Can you work these out from the model? Positions are in its coordinate system, mm. A direction names the side the tool comes from. Give positions to 0.01 mm unless a question says otherwise; leave off trailing zeros. Loops run counter-clockwise (first coordinate to the right, second up) from the corner with the lowest first, then second, coordinate; pieces in that order, holes last. Notation, with made-up numbers: M 5.5,7.5 L 11.5,7.5 A25 cw 11.5,44.5 Z; hole C 50,-31.75 d6. An arc over 180 degrees is marked long. Answer as a JSON object with one key per item and string values.
```python
from build123d import *

# Parameters (mm, degrees)
SKETCH1_W           = 154
SKETCH1_H           = 51
SKETCH1_R           = 1.7
BOSS_EXTRUDE1_DEPTH = 4
SKETCH2_W           = 127
SKETCH2_H           = 28
BOSS_EXTRUDE2_DEPTH = 10


with BuildPart() as part:
    # Sketch1 → Boss-Extrude1 (new body)
    with BuildSketch(Plane(origin=(0, 0, 0), x_dir=(1, 0, 0), z_dir=(0, 1, 0))):
        with Locations((77, 25.5)):
            Rectangle(SKETCH1_W, SKETCH1_H)
        with Locations(Location((77, 25.5, 0), (0, 0, 270))):
            Circle(SKETCH1_R, mode=Mode.SUBTRACT)
        with Locations(Location((13.4, 25.5, 0), (0, 0, 270))):
            Circle(SKETCH1_R, mode=Mode.SUBTRACT)
        with Locations(Location((140.6, 25.5, 0), (0, 0, 90))):
            Circle(SKETCH1_R, mode=Mode.SUBTRACT)
    extrude(amount=BOSS_EXTRUDE1_DEPTH)

    # Sketch2 → Boss-Extrude2 (add)
    with BuildSketch(Plane(origin=(0, 4, 0), x_dir=(1, 0, 0), z_dir=(0, 1, 0))):
        with Locations((63.5, 27)):
            Rectangle(SKETCH2_W, SKETCH2_H)
    extrude(amount=BOSS_EXTRUDE2_DEPTH)


solid = part.part
```
1) Suppose I cut it at B-B, the plane x = 140.6. Write out the boundary of the cut face in (y, z).
Answer list:
{"outline": "M 0,-51 L 4,-51 L 4,-27.2 L 0,-27.2 Z; M 0,-23.8 L 4,-23.8 L 4,0 L 0,0 Z"}
2) Suppose I cut it at C-C, the plane x = 77. Write out the boundary of the cut face in (y, z), and give its area (3 significant figures).
Answer list:
{"outline": "M 0,-51 L 4,-51 L 4,-41 L 14,-41 L 14,-13 L 4,-13 L 4,0 L 0,0 L 0,-23.8 L 4,-23.8 L 4,-27.2 L 0,-27.2 Z", "area": "470 mm^2"}
3) Suppose I cut it at A-A, the plane z = -25.5. Write out the boundary of the cut face in (x, y), and give its area (3 significant figures).
Answer list:
{"outline": "M 0,0 L 11.7,0 L 11.7,4 L 15.1,4 L 15.1,0 L 75.3,0 L 75.3,4 L 78.7,4 L 78.7,0 L 138.9,0 L 138.9,4 L 127,4 L 127,14 L 0,14 Z; M 142.3,0 L 154,0 L 154,4 L 142.3,4 Z", "area": "1,850 mm^2"}
4) If we mould it in two halves opening along Z, with no side actions, what happens to faces 1 (the flat face through (63, 9, -13)), 2 (the flat face through (154, 2, -25)), 3 (the cylindrical face through (14.833, 1.972, -24.586))? For each: +Z half, -Z half, draft (parallel to the pull), parting line (faces both ways), or undercut.
Answer list:
{"face 1": "+Z half", "face 2": "draft", "face 3": "undercut"}
5) Please list where these lines run through material, in increasing order: line 1 along X through (y, z) = (1.7, -25.5); line 2 along Z through (x, y) = (140.6, 2.05); line 3 along Z through (x, y) = (75.5, 7). Write a range as from..to.
Answer list:
{"line 1": "0..11.7, 15.1..75.3, 78.7..138.9, 142.3..154", "line 2": "-51..-27.2, -23.8..0", "line 3": "-41..-13"}
6) Will these pins go through, and if not, where does the flat tip stop? pin 1 Ø1 at (x, y) = (100, 7.5) entering from +Z; pin 2 Ø1.5 at (x, y) = (21, 10) entering from -Z; pin 3 Ø2.5 at (x, z) = (77, -25.5) entering from -Y.
Answer list:
{"pin 1": "z = -13", "pin 2": "z = -41", "pin 3": "y = 4"}
7) For faces 4 (the flat face through (77, 4, -26)), 5 (the flat face through (63, 9, -41)), 6 (the flat face through (76, 2, -51)), 7 (the cylindrical face through (139.167, 1.972, -26.414)), 8 (the flat face through (127, 9, -27)), which set-ups out of +Z, -Z, +X, -X, +Y, -Y let a thin tool reach every point of the face, with its end or its side?
Answer list:
{"face 4": "-Y", "face 5": "-Z, +X, -X, +Y", "face 6": "-Z, +X, -X, +Y, -Y", "face 7": "+Y, -Y", "face 8": "+Z, -Z, +X, +Y"}
8) Suppose I cut it at D-D, the plane z = -39. Write out the boundary of the cut face in (x, y).
Answer list:
{"outline": "M 0,0 L 154,0 L 154,4 L 127,4 L 127,14 L 0,14 Z"}
